The model under review builds one solid part; all positions refer to its coordinate system, in mm. Give positions to 0.01 mm unless a question says otherwise; leave off trailing zeros. Order: outer loops, then holes, each group sorted by start corner. A loop starts at its lowest first (then second) coordinate and runs counter-clockwise, first axis right, second up. Notation, with made-up numbers: (56, -28) - (63, -28) arc R26 ccw to (63, 0) - close; hole circle Ø10 at (-4.5, -12.75). An arc over 180 degrees is marked (long way). Put each result on its own line as item: value.
```python
from build123d import *

# Parameters (mm, degrees)
SCHIZZO1_R                   = 5
SCHIZZO1_W                   = 10
SCHIZZO1_H                   = 4
ESTRUSIONE_ESTRUSIONE3_DEPTH = 4


with BuildPart() as part:
    # Schizzo1 → Estrusione-Estrusione3 (new body)
    with BuildSketch(Plane.XY):
        with BuildLine():
            Line((0, 0), (700, 0))
            Line((700, 0), (700, 30))
            Line((700, 30), (700, 73))
            ThreePointArc((700, 73), (697.949747468, 77.949747468), (693, 80))
            Line((693, 80), (654.193736081, 80))
            ThreePointArc((654.193736081, 80), (652.382002765, 79.761480784), (650.693736081, 79.062177826))
            Line((650.693736081, 79.062177826), (581.959107885, 39.378221735))
            ThreePointArc((581.959107885, 39.378221735), (565.076441043, 32.38519216), (546.959107885, 30))
            Line((546.959107885, 30), (0, 30))
            Line((0, 30), (0, 0))
        make_face()
        with Locations((200, 15)):
            Circle(SCHIZZO1_R, mode=Mode.SUBTRACT)
        with Locations((150, 23)):
            Rectangle(SCHIZZO1_W, SCHIZZO1_H, mode=Mode.SUBTRACT)
        with Locations((50, 23)):
            Rectangle(SCHIZZO1_W, SCHIZZO1_H, mode=Mode.SUBTRACT)
        with Locations((250, 23)):
            Rectangle(SCHIZZO1_W, SCHIZZO1_H, mode=Mode.SUBTRACT)
        with Locations((350, 23)):
            Rectangle(SCHIZZO1_W, SCHIZZO1_H, mode=Mode.SUBTRACT)
        with Locations((450, 23)):
            Rectangle(SCHIZZO1_W, SCHIZZO1_H, mode=Mode.SUBTRACT)
        with Locations((550, 23)):
            Rectangle(SCHIZZO1_W, SCHIZZO1_H, mode=Mode.SUBTRACT)
        with Locations((650, 23)):
            Rectangle(SCHIZZO1_W, SCHIZZO1_H, mode=Mode.SUBTRACT)
        with BuildLine():
            Line((690, 63), (690, 37))
            ThreePointArc((690, 37), (687.949747468, 32.050252532), (683, 30))
            Line((683, 30), (611.839907009, 30))
            ThreePointArc((611.839907009, 30), (605.078426225, 35.188266684), (608.339907009, 43.062177826))
            Line((608.339907009, 43.062177826), (653.373228005, 69.062177826))
            ThreePointArc((653.373228005, 69.062177826), (655.06149469, 69.761480784), (656.873228005, 70))
            Line((656.873228005, 70), (683, 70))
            ThreePointArc((683, 70), (687.949747468, 67.949747468), (690, 63))
        make_face(mode=Mode.SUBTRACT)
    extrude(amount=ESTRUSIONE_ESTRUSIONE3_DEPTH)


solid = part.part
```
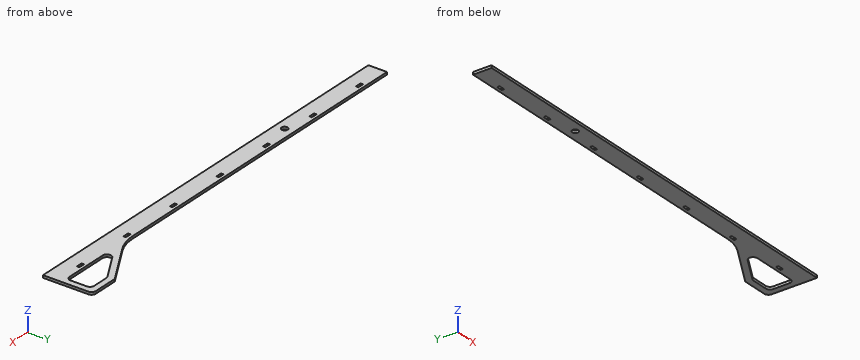
(1) Wall thickness on L1, parallel to Y at x = 346, z = 1.3; L2, parallel to Y at x = 200, z = 2.2; L3, parallel to Y at x = 654, z = 0.7: over which ranges is each line inside the solid? List them lowest first.
The answers:
L1: 0 to 21, 25 to 30
L2: 0 to 10, 20 to 30
L3: 0 to 21, 25 to 30, 69.38 to 80
(2) Take a section at A-A, the plane y = 55. Write out the cut boundary in (x, z).
The answers:
outline: (609.02, 0) - (629.02, 0) - (629.02, 4) - (609.02, 4) - close; (690, 0) - (700, 0) - (700, 4) - (690, 4) - close
(3) Clearance check with a flat-ended pin moving along its axis: pin 1 Ø1.2 at (x, z) = (147.5, 3) entering from +Y. State where the tip first meets the part, or that it passes through.
The answers:
pin 1: y = 30
(4) Take a section at C-C, the plane x = 275. Write out the cut boundary in (y, z), then the cut area to 3 significant figures.
The answers:
outline: (0, 0) - (30, 0) - (30, 4) - (0, 4) - close
area: 120 mm^2
(5) Take a section at B-B, the plane z = 3. Count the separate pieces of the cut face and the enclosed holes in it, then the cut area to 3 significant figures.
The answers:
separate pieces: 1
enclosed holes: 9
area: 22,600 mm^2
(6) Take a section at D-D, the plane x = 592.5. Write out the cut boundary in (y, z).
The answers:
outline: (0, 0) - (45.46, 0) - (45.46, 4) - (0, 4) - close
